from build123d import *

# Parameters (mm, degrees)
SKETCH3_W            = 4.5
SKETCH3_H            = 48
SKETCH3_W_2          = 8
SKETCH3_H_2          = 60
BOSS_EXTRUDE2_DEPTH  = 4.5
SKETCH4_W            = 5
SKETCH4_H            = 41
BOSS_EXTRUDE3_DEPTH  = 5.5
SKETCH6_W            = 2
SKETCH6_H            = 60
BOSS_EXTRUDE4_DEPTH  = 5.5
SKETCH7_W            = 41
SKETCH7_H            = 5.5
BOSS_EXTRUDE5_DEPTH  = 4
M2_CLEARANCE_SLOT1_D = 2.4


with BuildPart() as part:
    # Sketch3 → Boss-Extrude2 (new body)
    with BuildSketch(Plane(origin=(0, 0, 0), x_dir=(1, 0, 0), z_dir=(0, 1, 0))):
        with Locations((-8.027777778, 26.190445059)):
            Rectangle(SKETCH3_W, SKETCH3_H)
        with Locations((-1.777777778, 26.190445059)):
            Rectangle(SKETCH3_W_2, SKETCH3_H_2)
    extrude(amount=BOSS_EXTRUDE2_DEPTH)

    # Sketch4 → Boss-Extrude3 (add)
    with BuildSketch(Plane(origin=(0, 4.5, 0), x_dir=(1, 0, 0), z_dir=(0, 1, 0))):
        with Locations((-8.23478156, 26.190445059)):
            Rectangle(SKETCH4_W, SKETCH4_H)
    extrude(amount=BOSS_EXTRUDE3_DEPTH)

    # Sketch6 → Boss-Extrude4 (add)
    with BuildSketch(Plane(origin=(0, 4.5, 0), x_dir=(1, 0, 0), z_dir=(0, 1, 0))):
        with Locations((-4.777777778, 26.190445059)):
            Rectangle(SKETCH6_W, SKETCH6_H)
    extrude(amount=BOSS_EXTRUDE4_DEPTH)

    # Sketch7 → Boss-Extrude5 (add)
    with BuildSketch(Plane.ZY.offset(10.73478156)):
        with Locations((-26.190445059, 7.25)):
            Rectangle(SKETCH7_W, SKETCH7_H)
    extrude(amount=BOSS_EXTRUDE5_DEPTH)

    # M2 Clearance Slot1 (through all)
    with Locations(Plane(origin=(-24.675307519, 4.5, -134.803183417), x_dir=(1, 0, 0), z_dir=(0, 1, 0))):
        with Locations((23.920998694, -125.399645606), (23.920998694, -92.291639463)):
            Hole(M2_CLEARANCE_SLOT1_D / 2)


solid = part.part
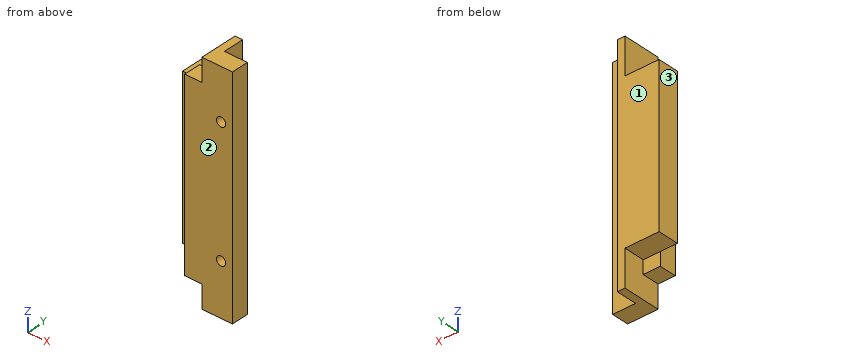
Here's how the part is built. I have some questions about the finished solid (model axes, mm). Face numbers are marked on the shaded views. Round coordinates to 2 decimals unless told otherwise and drop trailing zeros. Write each loop counter-clockwise with the first axis right and the second up, starting at its lowest first coordinate (ties: lowest second). Pieces come first, ordered by that corner, then holes.
1. Suppose I cut it at B-B (x = -8.25). List the corners of the cut face in (y, z) for me, and give its area (4 significant figures).
2. If we mould it in two halves opening along Y, with no side actions, what happens to the marked faces 1, 2 and 3? For each: released by +Y, released by -Y, zero draft, split by the parting line, or undercut.
3. Suppose I cut it at A-A (z = -29). List the corners of the cut face in (x, y) for me.
4. Suppose I cut it at D-D (x = -1). List the corners of the cut face in (y, z) for me.
5. Suppose I cut it at C-C (y = 1.75). List the corners of the cut face in (x, z) for me, and give its area (3 significant figures).
6. Will these pins go through, and if not, where does the flat tip stop? pin 1 Ø3 at (y, z) = (3, -49.5) entering from -X; pin 2 Ø4 at (y, z) = (3.5, -17.5) entering from -X; pin 3 Ø1.6 at (y, z) = (7.5, -23) entering from +X; pin 4 Ø1.8 at (x, z) = (-8, -48) entering from +Y.
7. I need wall thicknesses on L1, parallel to Z at x = -0.75, y = 3.5; L2, parallel to Y at x = -13.25, z = -29.5; L3, parallel to X at y = 8.5, z = -34. Which ranges of each line are inside material? Lowest first, please.
Answer sheet:
1. outline: (0, -50.19) - (4.5, -50.19) - (4.5, -46.69) - (10, -46.69) - (10, -5.69) - (4.5, -5.69) - (4.5, -2.19) - (0, -2.19) - close
1. area: 441.5 mm2
2. face 1: released by +Y
2. face 2: released by -Y
2. face 3: zero draft
3. outline: (-14.73, 4.5) - (-10.28, 4.5) - (-10.28, 0) - (2.22, 0) - (2.22, 4.5) - (-3.78, 4.5) - (-3.78, 10) - (-14.73, 10) - close
4. outline: (0, -56.19) - (4.5, -56.19) - (4.5, -43.69) - (0, -43.69) - close; (0, -41.34) - (4.5, -41.34) - (4.5, -10.58) - (0, -10.58) - close; (0, -8.23) - (4.5, -8.23) - (4.5, 3.81) - (0, 3.81) - close
5. outline: (-10.28, -50.19) - (-5.78, -50.19) - (-5.78, -56.19) - (2.22, -56.19) - (2.22, 3.81) - (-5.78, 3.81) - (-5.78, -2.19) - (-10.28, -2.19) - close; hole circle Ø2.4 at (-0.75, -42.51); hole circle Ø2.4 at (-0.75, -9.4)
5. area: 687 mm2
6. pin 1: stops at x = -10.28
6. pin 2: stops at x = -14.73
6. pin 3: stops at x = -3.78
6. pin 4: stops at y = 4.5
7. L1: z = -56.19 to -43.71, -41.31 to -10.6, -8.2 to 3.81
7. L2: y = 4.5 to 10
7. L3: x = -14.73 to -3.78
